```python
from build123d import *

# Parameters (mm, degrees)
SKETCH_R      = 4
PAD_DEPTH     = 6.5
SKETCH001_R   = 11
SKETCH001_R_2 = 6
POCKET_DEPTH  = 2
FILLET_R      = 3
FILLET001_R   = 1
SKETCH002_R   = 2.3
HOLE_DEPTH    = 25


with BuildPart() as part:
    # Sketch → Pad (new body, symmetric)
    with BuildSketch(Plane.XZ):
        with BuildLine():
            ThreePointArc((13.688033, 2.939003), (0, 14), (-13.688033, 2.939003))
            Line((-13.688033, 2.939003), (-15.5, -5.5))
            Line((-15.5, -5.5), (-27.5, -5.5))
            Line((-27.5, -5.5), (-27.5, -15))
            Line((-27.5, -15), (27.5, -15))
            Line((27.5, -15), (27.5, -5.5))
            Line((27.5, -5.5), (15.5, -5.5))
            Line((15.5, -5.5), (13.688033, 2.939003))
        make_face()
        Circle(SKETCH_R, mode=Mode.SUBTRACT)
    extrude(amount=PAD_DEPTH, both=True)

    # Sketch001 (on Face11 of Pad) → Pocket (cut)
    with BuildSketch(Plane.XZ.offset(6.5)):
        Circle(SKETCH001_R)
        Circle(SKETCH001_R_2, mode=Mode.SUBTRACT)
    pocket = extrude(amount=-POCKET_DEPTH, mode=Mode.SUBTRACT)

    # Mirrored: Pocket across XZ
    add(pocket.mirror(Plane.XZ), mode=Mode.SUBTRACT)

    # Fillet
    fillet_edges = [part.edges().sort_by_distance(p)[0] for p in [
        (15.5, 0, -5.5),
        (-15.5, 0, -5.5),
    ]]
    fillet(fillet_edges, radius=FILLET_R)

    # Fillet001
    fillet001_edges = [part.edges().sort_by_distance(p)[0] for p in [
        (-27.5, 0, -5.5),
        (27.5, 0, -5.5),
    ]]
    fillet(fillet001_edges, radius=FILLET001_R)

    # Sketch002 (on Face13 of Fillet001) → Hole (cut)
    with BuildSketch(Plane(origin=(0, 0, -5.5), x_dir=(-1, 0, 0), z_dir=(0, 0, 1))):
        with Locations((-21, 0)):
            Circle(SKETCH002_R)
        with Locations((21, 0)):
            Circle(SKETCH002_R)
    extrude(amount=-HOLE_DEPTH, mode=Mode.SUBTRACT)


solid = part.part
```
Input: part model. Units: mm. Frame: model coordinates. A direction names the side the tool comes from. Give positions to 0.01 mm unless a question says otherwise; leave off trailing zeros. Order: outer loops, then holes, each group sorted by start corner. A loop starts at its lowest first (then second) coordinate and runs counter-clockwise, first axis right, second up. Notation, with made-up numbers: (87.25, 41.5) - (142.25, 41.5) arc R7 cw to (142.25, 46.5) - close; hole circle Ø2 at (57, 71.25). An arc over 180 degrees is marked (long way). Put each result on its own line as item: value.
Item 1: Section query D-D, the plane z = 0. Return loops of the section in (x, y), then the cut area to 3 significant figures.
Found:
outline: (-14.32, -6.5) - (-11, -6.5) - (-11, -4.5) - (-6, -4.5) - (-6, -6.5) - (-4, -6.5) - (-4, 6.5) - (-6, 6.5) - (-6, 4.5) - (-11, 4.5) - (-11, 6.5) - (-14.32, 6.5) - close; (4, -6.5) - (6, -6.5) - (6, -4.5) - (11, -4.5) - (11, -6.5) - (14.32, -6.5) - (14.32, 6.5) - (11, 6.5) - (11, 4.5) - (6, 4.5) - (6, 6.5) - (4, 6.5) - close
area: 228 mm^2
Item 2: Draft query along Z for faces 4 (the cylindrical face through (18.806, -0.691, -10.183)), 5 (the cylindrical face through (-6, 6, 0)), 6 (the flat face through (-14.33, -0.09, -0.05)), 7 (the flat face through (5, 4.5, -5)). Return one class per face: +Z half, -Z half, draft (parallel to the pull), parting line (faces both ways), or undercut.
Found:
face 4: draft
face 5: undercut
face 6: +Z half
face 7: undercut
Item 3: Section query A-A, the plane x = 21. Return loops of the section in (y, z), then the cut area to 3 significant figures.
Found:
outline: (-6.5, -15) - (-2.3, -15) - (-2.3, -5.5) - (-6.5, -5.5) - close; (2.3, -15) - (6.5, -15) - (6.5, -5.5) - (2.3, -5.5) - close
area: 79.8 mm^2
Item 4: Contact query for flat-ended pins moving along their axis: pin 1 (5 mm diameter, centred on x = 10, y = 0, fed in from +Z); pin 2 (6 mm diameter, centred on y = -5, z = -2, fed in from +X); pin 3 (1.5 mm diameter, centred on y = -2, z = -0.5, fed in from -X). Output: stop coordinate, or through.
Found:
pin 1: stops at z = 11.82
pin 2: stops at x = 16.27
pin 3: stops at x = -14.59
Item 5: Access query for faces 1 (the flat face through (5, -4.5, -5)), 2 (the cylindrical face through (-2.38, 5.51, -10.74)), 3 (the flat face through (23, -2, -5.5)). Directions: +Z, -Z, +X, -X, +Y, -Y. A direction counts if a zero-diameter tool reaches every point of the face in a straight line with its end or side. Return the directions, or none.
Found:
face 1: -Y
face 2: +Y
face 3: +Z, +X, +Y, -Y
Item 6: Ray query, L1, parallel to Z at x = 0, y = -5.3; L2, parallel to X at y = 0, z = -9.5; L3, parallel to Y at x = 21, z = -9. Return the intervals inside material, ascending. Write a range as from..to.
Found:
L1: z = -15..-11, -6..-4, 4..6, 11..14
L2: x = -27.5..-23.3, -18.7..18.7, 23.3..27.5
L3: y = -6.5..-2.3, 2.3..6.5
Item 7: Section query C-C, the plane y = 3. Return loops of the section in (x, z).
Found:
outline: (-27.5, -15) - (27.5, -15) - (27.5, -6.5) arc R1 ccw to (26.5, -5.5) - (17.92, -5.5) arc R3 cw to (14.99, -3.13) - (13.69, 2.94) arc R14 ccw to (-13.69, 2.94) - (-14.99, -3.13) arc R3 cw to (-17.92, -5.5) - (-26.5, -5.5) arc R1 ccw to (-27.5, -6.5) - close; hole circle Ø8 at (0, 0)
Item 8: Section query B-B, the plane y = 0. Return loops of the section in (x, z).
Found:
outline: (-27.5, -15) - (-23.3, -15) - (-23.3, -5.5) - (-26.5, -5.5) arc R1 ccw to (-27.5, -6.5) - close; (-18.7, -15) - (18.7, -15) - (18.7, -5.5) - (17.92, -5.5) arc R3 cw to (14.99, -3.13) - (13.69, 2.94) arc R14 ccw to (-13.69, 2.94) - (-14.99, -3.13) arc R3 cw to (-17.92, -5.5) - (-18.7, -5.5) - close; (23.3, -15) - (27.5, -15) - (27.5, -6.5) arc R1 ccw to (26.5, -5.5) - (23.3, -5.5) - close; hole circle Ø8 at (0, 0)
